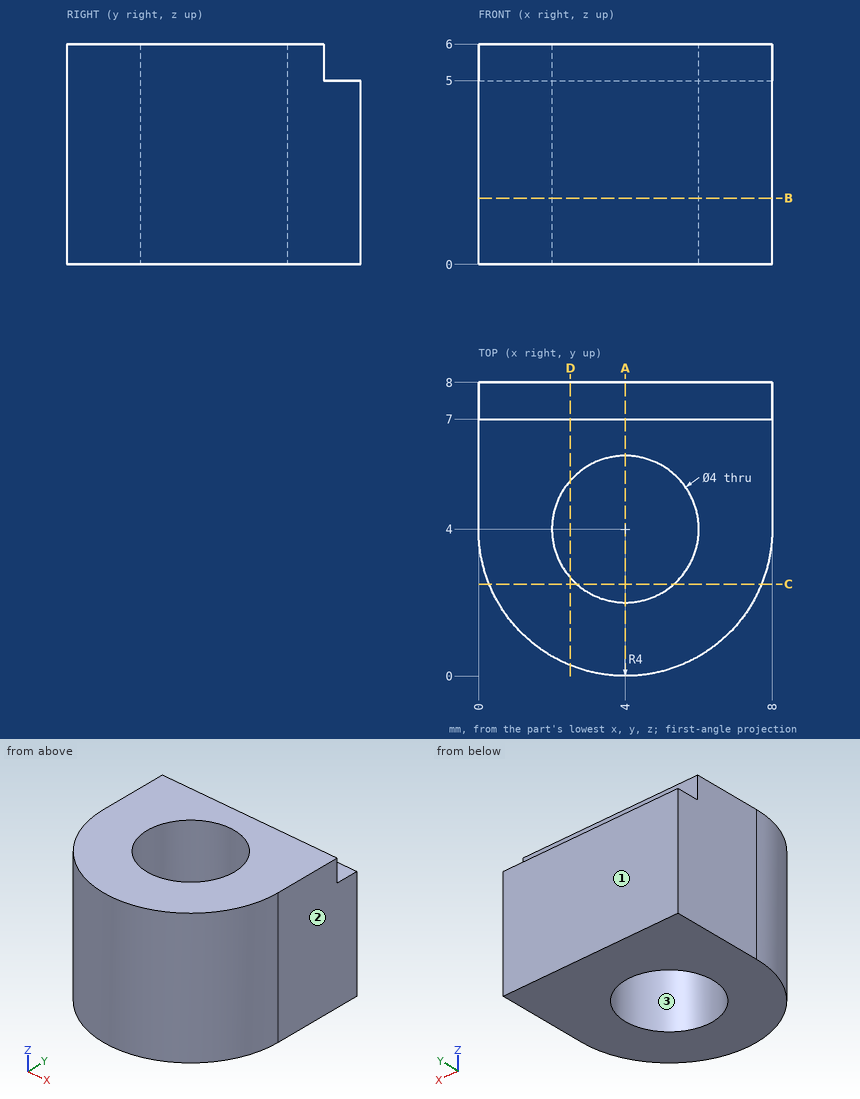
Design review of the part shown in the three views and the two pictorial views. Dimensions are in mm from the part's minimum x, y and z. Round coordinates to 2 decimals unless told otherwise and drop trailing zeros. Loops run counter-clockwise (first coordinate to the right, second up) from the corner with the lowest first, then second, coordinate; pieces in that order, holes last. Notation, with made-up numbers: (-6, -30) -> (49, -30) arc R38 ccw to (49, 9) -> close; hole circle Ø9 at (4, 63). An arc over 180 degrees is marked (long way). Answer as CSV lines item,"result".
1) Draft analysis for pull direction X (two halves, no side actions). For the marked faces 1, 2 and 3, state which applies: pulls with the +X half, pulls with the -X half, needs draft (parallel to the pull), parting line crosses it, or undercut.
Geometry results:
face 1,"needs draft"
face 2,"pulls with the +X half"
face 3,"undercut"
2) Add section D-D on x = 2.5. Write out the cut boundary in (y, z), plus the area to 3 significant figures.
Geometry results:
outline,"(0.29, 0) -> (2.68, 0) -> (2.68, 6) -> (0.29, 6) -> close; (5.32, 0) -> (8, 0) -> (8, 5) -> (7, 5) -> (7, 6) -> (5.32, 6) -> close"
area,"29.4 mm²"
3) Add section B-B on z = 1.8. Write out the cut boundary in (x, y), plus the area to 3 significant figures.
Geometry results:
outline,"(0, 4) arc R4 ccw to (8, 4) -> (8, 8) -> (0, 8) -> close; hole circle Ø4 at (4, 4)"
area,"44.6 mm²"
4) To check wall thickness, follow line 1 along Y through (x, z) = (4, 4.35); line 2 along X through (y, z) = (4.5, 4.3); line 3 along X through (y, z) = (5.75, 4.5). State the ranges of each line that lie inside material, in increasing order. Write a range as from..to.
Geometry results:
line 1,"y = 0..2, 6..8"
line 2,"x = 0..2.06, 5.94..8"
line 3,"x = 0..3.03, 4.97..8"
5) For P1, Ø0.8, axis at x = 3, y = 7.5, coming from the +Z side; P2, Ø1.5, axis at x = 6.5, z = 4.5, coming from the -Y side; P3, Ø0.8, axis at x = 3, z = 5.5, coming from the +Y side, all flat-tipped, find the tip position at first contact; note any pin that passes through.
Geometry results:
P1,"stops at z = 5"
P2,"stops at y = 0.4"
P3,"stops at y = 7"
6) Add section C-C on y = 2.5. Write out the cut boundary in (x, z), plus the area to 3 significant figures.
Geometry results:
outline,"(0.29, 0) -> (2.68, 0) -> (2.68, 6) -> (0.29, 6) -> close; (5.32, 0) -> (7.71, 0) -> (7.71, 6) -> (5.32, 6) -> close"
area,"28.6 mm²"
7) Add section A-A on x = 4. Write out the cut boundary in (y, z).
Geometry results:
outline,"(0, 0) -> (2, 0) -> (2, 6) -> (0, 6) -> close; (6, 0) -> (8, 0) -> (8, 5) -> (7, 5) -> (7, 6) -> (6, 6) -> close"
